CAD build for the part. Positions are in the model's coordinates, mm. Face numbers are marked on the shaded views. Give positions to 0.01 mm unless a question says otherwise; leave off trailing zeros. Write each loop counter-clockwise with the first axis right and the second up, starting at its lowest first coordinate (ties: lowest second). Pieces come first, ordered by that corner, then holes. Notation, with made-up numbers: (86, 1.5) -> (95, 1.5) arc R15 cw to (95, 27.5) -> close; hole circle Ø6 at (68, 44.25). An arc over 180 degrees is marked (long way). Answer as a JSON object with one key per item and string values.
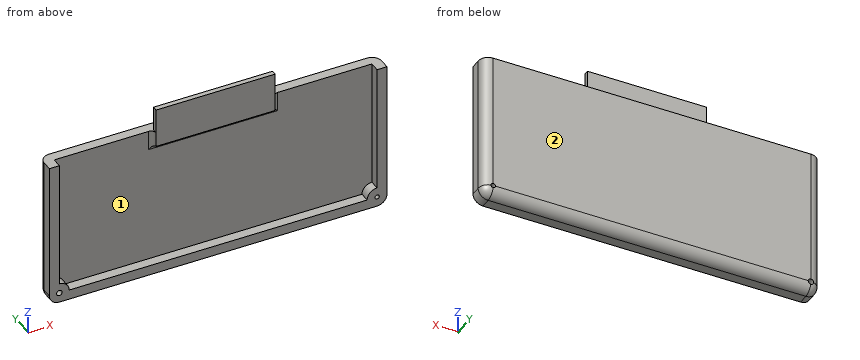
```python
from build123d import *

# Parameters (mm, degrees)
SKETCH1_W           = 170
SKETCH1_H           = 70
BOSS_EXTRUDE1_DEPTH = 90
FILLET2_R           = 5
SKETCH5_R           = 1.4
CUT_EXTRUDE2_DEPTH  = 12
CUT_EXTRUDE3_DEPTH  = 170
SKETCH7_W           = 158.942349138
SKETCH7_H           = 5
CUT_EXTRUDE4_DEPTH  = 70
SKETCH9_W           = 1.057650862
SKETCH9_H           = 5
SKETCH9_W_2         = 2.044997
CUT_EXTRUDE5_DEPTH  = 70
SKETCH12_W          = 5
SKETCH12_H          = 5
BOSS_EXTRUDE2_DEPTH = 75
SKETCH13_R          = 5
BOSS_EXTRUDE4_DEPTH = 5
SKETCH14_R          = 1.4
SKETCH14_R_2        = 1.115846917
CUT_EXTRUDE6_DEPTH  = 10
FILLET3_R           = 5
BOSS_EXTRUDE5_DEPTH = 2.5
SKETCH16_W          = 60
SKETCH16_H          = 2.5
BOSS_EXTRUDE6_DEPTH = 12.5
FILLET4_R           = 2.5


# Some blends are built 0.0001 mm under size
with BuildPart() as part:
    # Sketch1 → Boss-Extrude1 (new body)
    with BuildSketch(Plane.XY):
        Rectangle(SKETCH1_W, SKETCH1_H)
    extrude(amount=BOSS_EXTRUDE1_DEPTH)

    # Fillet2
    fillet2_edges = [part.edges().sort_by_distance(p)[0] for p in [
        (85, -35, 45),
        (-85, -35, 45),
        (-85, 35, 45),
        (85, 35, 45),
    ]]
    fillet(fillet2_edges, radius=FILLET2_R)

    # Sketch5 → Cut-Extrude2 (cut)
    with BuildSketch(Plane.XY.offset(90)):
        with Locations((-80, 30)):
            Circle(SKETCH5_R)
        with Locations((-80, -30)):
            Circle(SKETCH5_R)
        with Locations((80, 30)):
            Circle(SKETCH5_R)
        with Locations((80, -30)):
            Circle(SKETCH5_R)
    extrude(amount=-CUT_EXTRUDE2_DEPTH, mode=Mode.SUBTRACT)

    # Sketch6 → Cut-Extrude3 (cut)
    with BuildSketch(Plane.ZY.offset(85)):
        Polygon((0, 25), (0, -35), (90, -35), (90, 35), (75, 35), (75, 25), align=None)
    extrude(amount=-CUT_EXTRUDE3_DEPTH, mode=Mode.SUBTRACT)

    # Sketch7 → Cut-Extrude4 (cut)
    with BuildSketch(Plane.XY.offset(75)):
        with Locations((0.528825431, 27.5)):
            Rectangle(SKETCH7_W, SKETCH7_H)
    extrude(amount=-CUT_EXTRUDE4_DEPTH, mode=Mode.SUBTRACT)

    # Sketch9 → Cut-Extrude5 (cut)
    with BuildSketch(Plane.XY.offset(75)):
        with Locations((-79.471174569, 27.5)):
            Rectangle(SKETCH9_W, SKETCH9_H)
        with Locations((81.0224985, 27.5)):
            Rectangle(SKETCH9_W_2, SKETCH9_H)
    extrude(amount=-CUT_EXTRUDE5_DEPTH, mode=Mode.SUBTRACT)

    # Sketch12 → Boss-Extrude2 (add)
    with BuildSketch(Plane.XY.offset(75)):
        with Locations((82.5, 27.5)):
            Rectangle(SKETCH12_W, SKETCH12_H)
    extrude(amount=-BOSS_EXTRUDE2_DEPTH)

    # Sketch13 → Boss-Extrude4 (add)
    with BuildSketch(Plane(origin=(0, 25, 0), x_dir=(-1, 0, 0), z_dir=(0, -1, 0))):
        with Locations((-80, -5)):
            Circle(SKETCH13_R)
        with Locations((80, -5)):
            Circle(SKETCH13_R)
    extrude(amount=-BOSS_EXTRUDE4_DEPTH)

    # Sketch14 → Cut-Extrude6 (cut)
    with BuildSketch(Plane.XZ.offset(-25)):
        with Locations((-80, 5)):
            Circle(SKETCH14_R)
        with Locations((80, 5)):
            Circle(SKETCH14_R_2)
    extrude(amount=-CUT_EXTRUDE6_DEPTH, mode=Mode.SUBTRACT)

    # Fillet3
    # the kernel refuses this fillet: 5 mm, written as the material it takes off along each edge
    with BuildSketch(Plane(origin=(-80, 35, 0), x_dir=(0, 0, 1), z_dir=(1, 0, 0))) as fillet3_piece_1:
        with BuildLine():
            CenterArc((FILLET3_R, FILLET3_R), FILLET3_R, 180, 90)
            Line((0, FILLET3_R), (0, 0))
            Line((0, 0), (FILLET3_R, 0))
        make_face()
    extrude(amount=160, mode=Mode.SUBTRACT)
    with BuildSketch(Plane(origin=(80, 30, 0), x_dir=(0, 1, 0), z_dir=(-1, 0, 0))) as fillet3_piece_2:
        with BuildLine():
            CenterArc((5 - FILLET3_R, -FILLET3_R), FILLET3_R, 0, 90)
            Line((5, -FILLET3_R), (5, 0))
            Line((5, 0), (5 - FILLET3_R, 0))
        make_face()
    revolve(axis=Axis((80, 30, 0), (0, 0, -1)), revolution_arc=90, mode=Mode.SUBTRACT)
    with BuildSketch(Plane(origin=(85, 30, 0), x_dir=(-1, 0, 0), z_dir=(0, -1, 0)), Plane(origin=(-85, 12.5, 0), x_dir=(1, 0, 0), z_dir=(0, 1, 0))) as fillet3_piece_3:
        with BuildLine():
            CenterArc((FILLET3_R, -FILLET3_R), FILLET3_R, 90, 90)
            Line((0, -FILLET3_R), (0, 0))
            Line((0, 0), (FILLET3_R, 0))
        make_face()
    extrude(amount=17.5, mode=Mode.SUBTRACT)
    with BuildSketch(Plane(origin=(-80, 30, 0), x_dir=(0, 1, 0), z_dir=(1, 0, 0))) as fillet3_piece_4:
        with BuildLine():
            CenterArc((5 - FILLET3_R, FILLET3_R), FILLET3_R, 270, 90)
            Line((5, FILLET3_R), (5, 0))
            Line((5, 0), (5 - FILLET3_R, 0))
        make_face()
    revolve(axis=Axis((-80, 30, 0), (0, 0, 1)), revolution_arc=90, mode=Mode.SUBTRACT)

    # Sketch15 → Boss-Extrude5 (add)
    with BuildSketch(Plane.XZ.offset(-30)):
        Polygon((0, 75), (30, 75), (30, 67.5), (-30, 67.5), (-30, 75), align=None)
    extrude(amount=BOSS_EXTRUDE5_DEPTH)

    # Sketch16 → Boss-Extrude6 (add)
    with BuildSketch(Plane.XY.offset(75)):
        with Locations((0, 28.75)):
            Rectangle(SKETCH16_W, SKETCH16_H)
    extrude(amount=BOSS_EXTRUDE6_DEPTH)

    # Fillet4
    fillet4_edges = [part.edges().sort_by_distance(p)[0] for p in [
        (-30, 30, 71.25),
        (0, 30, 67.5),
        (30, 30, 71.25),
    ]]
    fillet(fillet4_edges, radius=FILLET4_R - 0.0001)  # a hair under: the kernel refuses the full size


solid = part.part
```
1) Wall check: probe 1 along X at (y, z) = (27, 34); probe 2 along Z at (x, y) = (-50.5, 25.75); probe 3 along Y at (x, z) = (45, 62). Give the ranges that are in metal, low to high.
Model answer:
{"probe 1": "x = -85 to -80, 80 to 85", "probe 2": "z = 0 to 5", "probe 3": "y = 30 to 35"}
2) Slice it at B-B (x = -42.5). List the corners of the cut face in (y, z).
Model answer:
{"outline": "(25, 0) -> (30, 0) arc R5 ccw to (35, 5) -> (35, 75) -> (30, 75) -> (30, 5) -> (25, 5) -> close"}
3) Slice it at C-C (y = 32.25). List the corners of the cut face in (x, z), then the cut area to 3 significant figures.
Model answer:
{"outline": "(-84.47, 5) arc R4.47 ccw to (-80, 0.53) -> (80, 0.53) arc R4.47 ccw to (84.47, 5) -> (84.47, 75) -> (-84.47, 75) -> close; hole circle Ø2.8 at (-80, 5); hole circle Ø2.23 at (80, 5)", "area": "12,600 mm2"}
4) Slice it at A-A (z = 54.5). List the corners of the cut face in (x, y), then the cut area to 3 significant figures.
Model answer:
{"outline": "(-85, 25) -> (-80, 25) -> (-80, 30) -> (80, 30) -> (80, 25) -> (85, 25) -> (85, 30) arc R5 ccw to (80, 35) -> (-80, 35) arc R5 ccw to (-85, 30) -> close", "area": "889 mm2"}
5) Pin check, flat tips, straight feed: pin 1 (2 mm diameter, centred on y = 32, z = 58, fed in from -X); pin 2 (4 mm diameter, centred on x = -19.5, y = 30.5, fed in from +Z); pin 3 (6 mm diameter, centred on x = -2.5, z = 83, fed in from +Y); pin 4 (1.2 mm diameter, centred on y = 28.5, z = 78, fed in from -X). Stop position of each tip, or through.
Model answer:
{"pin 1": "stops at x = -84.9", "pin 2": "stops at z = 87.5", "pin 3": "stops at y = 30", "pin 4": "stops at x = -30"}
6) Mould opens along X. For the marked faces 1 and 2 say: released by +X, released by -X, zero draft, split by the parting line, or undercut.
Model answer:
{"face 1": "undercut", "face 2": "zero draft"}
